Design review of the part built by this model. Coordinates are the model's own, in mm. Give positions to 0.01 mm unless a question says otherwise; leave off trailing zeros. Order: outer loops, then holes, each group sorted by start corner. A loop starts at its lowest first (then second) coordinate and runs counter-clockwise, first axis right, second up. Notation, with made-up numbers: (75, 34.25) -> (99, 34.25) arc R14 cw to (99, 58.25) -> close; hole circle Ø8 at (48.5, 62.5). An arc over 180 degrees is marked (long way). One line per item, written item: value. Start each with the question number.
1) Consider section B-B (y = -13.85). State the section outline as (x, z) points, plus the area to 4 significant figures.
2) Consider section A-A (x = 4). State the section outline as (y, z) points, plus the area to 3 significant figures.
3) Consider section C-C (x = 19). State the section outline as (y, z) points, plus the area to 3 significant figures.
4) For pin 1 (2.5 mm diameter, centred on x = 19, y = -34.09, fed in from +Z); pin 2 (0.8 mm diameter, centred on x = 10, z = 1, fed in from -Y); pin 3 (0.5 mm diameter, centred on y = -33.5, z = 1, fed in from +X), all flat-tipped, find the tip position at first contact; note any pin that passes through.
5) Consider section D-D (x = 10.5). State the section outline as (y, z) points, plus the area to 3 significant figures.
6) Wall thickness on line 1 along Y through (x, z) = (4, 1.2); line 2 along Y through (x, z) = (16.5, 0.8); line 3 along Y through (x, z) = (12.5, 0.9): over which ranges is each line inside the solid? List them lowest first. Write a range as from..to.
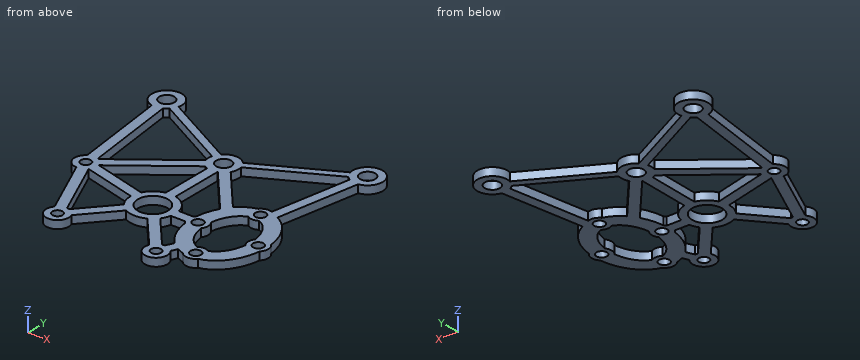
from build123d import *

# Parameters (mm, degrees)
SKETCH8_R           = 1
SKETCH8_R_2         = 1.500000001
SKETCH8_R_3         = 3
SKETCH8_R_4         = 1.5
SKETCH8_R_5         = 1.049999998
SKETCH8_R_6         = 1.05
BOSS_EXTRUDE1_DEPTH = 1.5875


with BuildPart() as part:
    # Sketch8 → Boss-Extrude1 (new body)
    with BuildSketch(Plane.XY):
        with BuildLine():
            Line((-13.086353998, -14.564609673), (1.796518672, -22.564153733))
            ThreePointArc((1.796518672, -22.564153733), (4.000000002, -21.6), (6.203481333, -22.564153733))
            Line((6.203481333, -22.564153733), (21.086354002, -14.564609673))
            ThreePointArc((21.086354002, -14.564609673), (25.651184859, -11.34528673), (24.491592476, -16.80944874))
            Line((24.491592476, -16.80944874), (21.594632818, -33.172177311))
            add(Edge.make_bspline(
                [(26.415943842, -40.678727885), (26.190074366, -38.784003898), (25.091906545, -35.832342913), (22.830851039, -33.788532272), (21.739107595, -33.238545613), (21.594632818, -33.172177311)],
                knots=[8.009475082, 8.009475082, 8.009475082, 8.009475082, 8.639379797, 9.032078879, 9.090955258, 9.090955258, 9.090955258, 9.090955258], degree=3))
            ThreePointArc((26.415943842, -40.678727885), (27.000000014, -42.091209061), (26.415943843, -43.503690238))
            add(Edge.make_bspline(
                [(20.516702098, -51.394901812), (21.03749091, -51.259926354), (22.533800563, -50.662395377), (25.091906547, -48.350075217), (26.190074368, -45.398414228), (26.415943843, -43.503690238)],
                knots=[6.474926491, 6.474926491, 6.474926491, 6.474926491, 6.675884389, 7.068583471, 7.698488187, 7.698488187, 7.698488187, 7.698488187], degree=3))
            ThreePointArc((20.516702098, -51.394901812), (19.000000019, -52.091209062), (17.483297936, -51.39490182))
            add(Edge.make_bspline(
                [(16.101578265, -50.861171127), (16.542577532, -51.091700443), (17.006966665, -51.271448649), (17.483297936, -51.39490182)],
                knots=[5.907641156, 5.907641156, 5.907641156, 5.907641156, 6.091444127, 6.091444127, 6.091444127, 6.091444127], degree=3))
            Line((16.101578265, -50.861171127), (15.561059424, -52.047023548))
            ThreePointArc((15.561059424, -52.047023548), (14.133861857, -55.693615173), (11.741313067, -52.593577485))
            Line((11.741313067, -52.593577485), (6.109164809, -46.066309546))
            ThreePointArc((6.109164809, -46.066309546), (4.000000002, -46.591209068), (1.890835194, -46.066309546))
            Line((1.890835194, -46.066309546), (-3.741313063, -52.593577485))
            ThreePointArc((-3.741313063, -52.593577485), (-6.139438128, -55.692810158), (-7.55392971, -52.038297803))
            Line((-7.55392971, -52.038297803), (-13.012969359, -39.900931113))
            ThreePointArc((-13.012969359, -39.900931113), (-15.09287941, -38.264638476), (-14.177523832, -35.78157513))
            Line((-14.177523832, -35.78157513), (-16.629703051, -16.783167924))
            ThreePointArc((-16.629703051, -16.783167924), (-17.592042406, -11.307284723), (-13.086353998, -14.564609673))
        make_face()
        with Locations((-12.927736722, -37.652546048)):
            Circle(SKETCH8_R, mode=Mode.SUBTRACT)
        with Locations((-15.999999999, -13.85)):
            Circle(SKETCH8_R_2, mode=Mode.SUBTRACT)
        with Locations((4.000000002, -42.091209068)):
            Circle(SKETCH8_R_3, mode=Mode.SUBTRACT)
        with Locations((4.000000002, -24.6)):
            Circle(SKETCH8_R_4, mode=Mode.SUBTRACT)
        with Locations((19.000000014, -34.091209062)):
            Circle(SKETCH8_R_5, mode=Mode.SUBTRACT)
        with Locations((25.000000014, -42.091209062)):
            Circle(SKETCH8_R_6, mode=Mode.SUBTRACT)
        with Locations((24.000000003, -13.85)):
            Circle(SKETCH8_R_4, mode=Mode.SUBTRACT)
        with Locations((19.000000014, -50.091209062)):
            Circle(SKETCH8_R_6, mode=Mode.SUBTRACT)
        with Locations((13.000000014, -42.091209062)):
            Circle(SKETCH8_R_5, mode=Mode.SUBTRACT)
        with Locations((13.815163294, -53.466300372)):
            Circle(SKETCH8_R, mode=Mode.SUBTRACT)
        with Locations((-5.81516329, -53.466300372)):
            Circle(SKETCH8_R, mode=Mode.SUBTRACT)
        with BuildLine():
            Line((-13.796518668, -15.885846268), (1.086354002, -23.885390328))
            ThreePointArc((1.086354002, -23.885390328), (1.002194363, -24.714722935), (1.149490441, -25.535197969))
            Line((1.149490441, -25.535197969), (-11.942202931, -35.629868826))
            ThreePointArc((-11.942202931, -35.629868826), (-12.066509782, -35.573895487), (-12.193978328, -35.52555319))
            Line((-12.193978328, -35.52555319), (-14.646157547, -16.527145984))
            ThreePointArc((-14.646157547, -16.527145984), (-14.192666478, -16.244482313), (-13.796518668, -15.885846268))
        make_face(mode=Mode.SUBTRACT)
        with BuildLine():
            Line((6.913646003, -23.885390328), (21.796518672, -15.885846268))
            ThreePointArc((21.796518672, -15.885846268), (22.137056458, -16.201476419), (22.522219684, -16.460778683))
            Line((22.522219684, -16.460778683), (19.730449721, -32.229370394))
            ThreePointArc((19.730449721, -32.229370394), (18.517890153, -32.150186115), (17.483297928, -32.787516314))
            add(Edge.make_bspline(
                [(17.483297928, -32.787516314), (16.962509109, -32.922491772), (15.727272297, -33.415766846), (14.665915712, -34.26639873), (14.116927694, -34.86100734)],
                knots=[3.333333835, 3.333333835, 3.333333835, 3.333333835, 3.534291735, 3.823410841, 3.823410841, 3.823410841, 3.823410841], degree=3))
            Line((14.116927694, -34.86100734), (6.60034411, -26.096065012))
            ThreePointArc((6.60034411, -26.096065012), (6.970318566, -25.020960368), (6.913646003, -23.885390328))
        make_face(mode=Mode.SUBTRACT)
        with BuildLine():
            Line((11.267949203, -41.091209067), (8.387482195, -41.091209067))
            ThreePointArc((8.387482195, -41.091209067), (7.181980517, -38.909228552), (5.000000002, -37.703726874))
            Line((5.000000002, -37.703726874), (5.000000002, -27.428427125))
            ThreePointArc((5.000000002, -27.428427125), (5.041188034, -27.41352581), (5.082154119, -27.398024744))
            Line((5.082154119, -27.398024744), (12.911091108, -36.527196283))
            add(Edge.make_bspline(
                [(12.911091108, -36.527196283), (12.211706609, -37.765848449), (11.760461262, -39.198939723), (11.584056161, -40.67872791)],
                knots=[4.064937043, 4.064937043, 4.064937043, 4.064937043, 4.556895536, 4.556895536, 4.556895536, 4.556895536], degree=3))
            ThreePointArc((11.584056161, -40.67872791), (11.412548353, -40.874657697), (11.267949203, -41.091209067))
        make_face(mode=Mode.SUBTRACT)
        with BuildLine():
            Line((11.267949213, -43.091209073), (8.387482194, -43.091209073))
            ThreePointArc((8.387482194, -43.091209073), (8.091394843, -43.964838767), (7.623388786, -44.759739322))
            Line((7.623388786, -44.759739322), (13.255537044, -51.287007261))
            ThreePointArc((13.255537044, -51.287007261), (13.496464731, -51.23898557), (13.741191761, -51.217516653))
            Line((13.741191761, -51.217516653), (14.450284347, -49.6618278))
            add(Edge.make_bspline(
                [(11.58405616, -43.503690213), (11.809925632, -45.398414212), (12.658784204, -47.679980557), (14.128913372, -49.352631306), (14.450284347, -49.6618278)],
                knots=[4.867882424, 4.867882424, 4.867882424, 4.867882424, 5.497787144, 5.65833174, 5.65833174, 5.65833174, 5.65833174], degree=3))
            ThreePointArc((11.58405616, -43.503690213), (11.412548358, -43.307760434), (11.267949213, -43.091209073))
        make_face(mode=Mode.SUBTRACT)
        with BuildLine():
            Line((-10.705156101, -37.20152807), (0, -40.029656258))
            ThreePointArc((0, -40.029656258), (1.242739245, -38.534874842), (3.000000002, -37.703726874))
            Line((3.000000002, -37.703726874), (3.000000002, -27.428427125))
            ThreePointArc((3.000000002, -27.428427125), (2.676302315, -27.292178381), (2.370745744, -27.119033657))
            Line((2.370745744, -27.119033657), (-10.705156101, -37.20152807))
        make_face(mode=Mode.SUBTRACT)
        with BuildLine():
            Line((-5.729930653, -51.217915307), (-11.15749378, -39.150532004))
            Line((-11.15749378, -39.150532004), (-0.497810837, -41.950860704))
            ThreePointArc((-0.497810837, -41.950860704), (-0.296617342, -43.428773795), (0.376611217, -44.759739322))
            Line((0.376611217, -44.759739322), (-5.255537039, -51.287007261))
            ThreePointArc((-5.255537039, -51.287007261), (-5.490888451, -51.239790585), (-5.729930653, -51.217915307))
        make_face(mode=Mode.SUBTRACT)
        with BuildLine():
            ThreePointArc((17.931899131, -35.782114294), (19.000000009, -36.091209062), (20.068100889, -35.782114299))
            add(Edge.make_bspline(
                [(23.417224995, -40.868579421), (23.351989797, -40.388373193), (23.059588765, -39.057302945), (22.112022209, -37.188969501), (20.925072461, -36.159009178), (20.236313774, -35.843572565), (20.068100889, -35.782114299)],
                knots=[8.033003045, 8.033003045, 8.033003045, 8.033003045, 8.246680716, 8.639379797, 9.032078879, 9.158456351, 9.158456351, 9.158456351, 9.158456351], degree=3))
            ThreePointArc((23.417224995, -40.868579421), (23.000000014, -42.091209063), (23.417224996, -43.313838704))
            add(Edge.make_bspline(
                [(20.068100897, -48.40030383), (20.23631378, -48.338845564), (20.925072464, -48.023408951), (22.112022209, -46.993448631), (23.059588765, -45.125115185), (23.351989798, -43.794044934), (23.417224996, -43.313838704)],
                knots=[6.549506919, 6.549506919, 6.549506919, 6.549506919, 6.675884389, 7.068583471, 7.461282552, 7.674960224, 7.674960224, 7.674960224, 7.674960224], degree=3))
            ThreePointArc((20.068100897, -48.40030383), (19.000000009, -48.091209062), (17.931899123, -48.400303835))
            add(Edge.make_bspline(
                [(14.582775013, -43.313838729), (14.648010212, -43.79404495), (14.940411244, -45.125115192), (15.887977797, -46.993448631), (17.074927547, -48.023408955), (17.763686236, -48.338845569), (17.931899123, -48.400303835)],
                knots=[4.891410394, 4.891410394, 4.891410394, 4.891410394, 5.105088062, 5.497787144, 5.890486225, 6.016863699, 6.016863699, 6.016863699, 6.016863699], degree=3))
            ThreePointArc((14.582775013, -43.313838729), (15.000000014, -42.091209063), (14.582775014, -40.868579396))
            add(Edge.make_bspline(
                [(17.931899131, -35.782114294), (17.763686241, -35.843572561), (17.07492755, -36.159009174), (15.887977797, -37.188969501), (14.940411245, -39.057302938), (14.648010213, -40.388373177), (14.582775014, -40.868579396)],
                knots=[9.691099567, 9.691099567, 9.691099567, 9.691099567, 9.817477042, 10.210176124, 10.602875206, 10.816552873, 10.816552873, 10.816552873, 10.816552873], degree=3))
        make_face(mode=Mode.SUBTRACT)
    extrude(amount=BOSS_EXTRUDE1_DEPTH)


solid = part.part
Checked values:
1. outline: (-19, 0) -> (-17.5, 0) -> (-17.5, 1.59) -> (-19, 1.59) -> close; (-14.5, 0) -> (-13, 0) -> (-13, 1.59) -> (-14.5, 1.59) -> close; (21, 0) -> (22.5, 0) -> (22.5, 1.59) -> (21, 1.59) -> close; (25.5, 0) -> (27, 0) -> (27, 1.59) -> (25.5, 1.59) -> close
1. area: 9.525 mm^2
2. outline: (-46.59, 0) -> (-45.09, 0) -> (-45.09, 1.59) -> (-46.59, 1.59) -> close; (-39.09, 0) -> (-26.1, 0) -> (-26.1, 1.59) -> (-39.09, 1.59) -> close; (-23.1, 0) -> (-21.6, 0) -> (-21.6, 1.59) -> (-23.1, 1.59) -> close
2. area: 25.4 mm^2
3. outline: (-52.09, 0) -> (-51.14, 0) -> (-51.14, 1.59) -> (-52.09, 1.59) -> close; (-49.04, 0) -> (-48.09, 0) -> (-48.09, 1.59) -> (-49.04, 1.59) -> close; (-36.09, 0) -> (-35.14, 0) -> (-35.14, 1.59) -> (-36.09, 1.59) -> close; (-33.04, 0) -> (-32.09, 0) -> (-32.09, 1.59) -> (-33.04, 1.59) -> close; (-17.39, 0) -> (-15.69, 0) -> (-15.69, 1.59) -> (-17.39, 1.59) -> close
3. area: 8.74 mm^2
4. pin 1: stops at z = 1.59
4. pin 2: stops at y = -51.04
4. pin 3: stops at x = 22.61
5. outline: (-51.15, 0) -> (-48.09, 0) -> (-48.09, 1.59) -> (-51.15, 1.59) -> close; (-43.09, 0) -> (-41.09, 0) -> (-41.09, 1.59) -> (-43.09, 1.59) -> close; (-33.72, 0) -> (-30.64, 0) -> (-30.64, 1.59) -> (-33.72, 1.59) -> close; (-21.96, 0) -> (-20.25, 0) -> (-20.25, 1.59) -> (-21.96, 1.59) -> close
5. area: 15.6 mm^2
6. line 1: y = -46.59..-45.09, -39.09..-26.1, -23.1..-21.6
6. line 2: y = -51.05..-47.47, -36.71..-33.13, -18.73..-17.03
6. line 3: y = -55.29..-50.41, -46.84..-43.01, -41.17..-37.34, -36.05..-32.98, -20.88..-19.18
